from build123d import *

# Parameters (mm, degrees)
F0_R     = 36.25
F0_R_2   = 25
F1_DEPTH = 2
F2_R     = 30
F2_R_2   = 32.5
F2_R_3   = 31
F3_DEPTH = 15
F4_R     = 0.5


with BuildPart() as f1:
    # F0 (on Top) → F1 (new body)
    with BuildSketch(Plane.XY):
        with Locations((0, 0.15434)):
            Circle(F0_R)
        Circle(F0_R_2, mode=Mode.SUBTRACT)
    extrude(amount=F1_DEPTH)

    # F2 (on face) → F3 (join)
    with BuildSketch(Plane.XY.offset(2)):
        Circle(F2_R)
        Circle(F2_R_2)
        Circle(F2_R_3, mode=Mode.SUBTRACT)
    extrude(amount=F3_DEPTH)

    # F4
    f4_edges = [f1.edges().sort_by_distance(p)[0] for p in [
        (-32.5, 0, 17),
        (-31, 0, 17),
    ]]
    fillet(f4_edges, radius=F4_R)


solid = f1.part
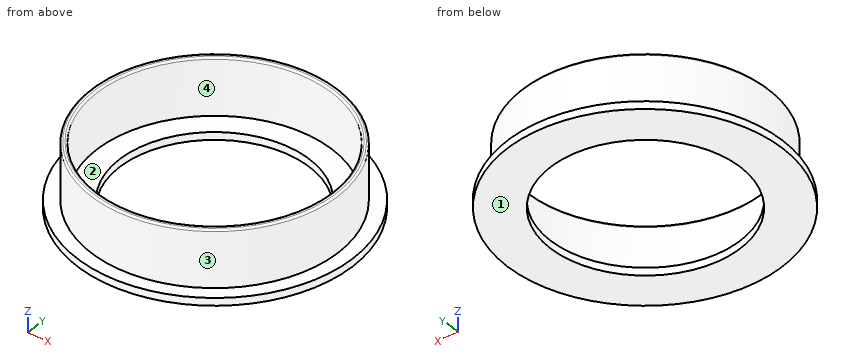
Verification items for the finished model (mm, model axes). Face numbers are marked on the shaded views. Round coordinates to 2 decimals unless told otherwise and drop trailing zeros. Order: outer loops, then holes, each group sorted by start corner. A loop starts at its lowest first (then second) coordinate and runs counter-clockwise, first axis right, second up. Notation, with made-up numbers: (-16.5, 84.5) -> (-3.5, 84.5) arc R18 ccw to (-3.5, 115.5) -> close; hole circle Ø4 at (61, -16.75). An arc over 180 degrees is marked (long way). Put each result on its own line as item: value.
1) Material ranges on line 1 (Y direction, x = 0, z = 6.5); line 2 (Y direction, x = 0, z = 0.6); line 3 (Z direction, x = 20, y = 18), recorded low to high.
Final values:
line 1: y = -32.5 to -31, 31 to 32.5
line 2: y = -36.1 to -25, 25 to 36.4
line 3: z = 0 to 2
2) Section check A-A (x = 0). Record the cut outline in (y, z), then the cut area to 3 significant figures.
Final values:
outline: (-36.1, 0) -> (-25, 0) -> (-25, 2) -> (-31, 2) -> (-31, 16.5) arc R0.5 ccw to (-31.5, 17) -> (-32, 17) arc R0.5 ccw to (-32.5, 16.5) -> (-32.5, 2) -> (-36.1, 2) -> close; (25, 0) -> (36.4, 0) -> (36.4, 2) -> (32.5, 2) -> (32.5, 16.5) arc R0.5 ccw to (32, 17) -> (31.5, 17) arc R0.5 ccw to (31, 16.5) -> (31, 2) -> (25, 2) -> close
area: 89.8 mm^2
3) Mould release check, pull along X, two halves, no side actions. Record for the marked faces 1, 2, 3 and 4: +X half, -X half, draft (parallel to the pull), parting line (faces both ways), or undercut.
Final values:
face 1: draft
face 2: undercut
face 3: parting line
face 4: undercut
4) Section check B-B (z = 7.5). Record the cut outline in (x, y).
Final values:
outline: circle Ø65 at (0, 0); hole circle Ø62 at (0, 0)
5) Depth check by flat-ended pin: pin 1 (10 mm diameter, centred on y = 1.5, z = 12, fed in from +X); pin 2 (8 mm diameter, centred on y = 20, z = 14.5, fed in from +X); pin 3 (1.5 mm diameter, centred on x = -25.5, z = 5.5, fed in from +Y). Enter the tip coordinate at first touch or a pass-through.
Final values:
pin 1: stops at x = 32.5
pin 2: stops at x = 28.29
pin 3: stops at y = 21.06
